Geometry check sheet. Reference: drawing and pictorial views, mm from the part's lowest x, y, z. Give positions to 0.01 mm unless a question says otherwise; leave off trailing zeros. Order: outer loops, then holes, each group sorted by start corner. A loop starts at its lowest first (then second) coordinate and runs counter-clockwise, first axis right, second up. Notation, with made-up numbers: M 35,36 L 45,36 A36 ccw 45,70 Z; hole C 89.25,-10.75 d7. An arc over 180 degrees is marked long. Use CSV: the item, a comma, the result in double quotes. Start each with the question number.
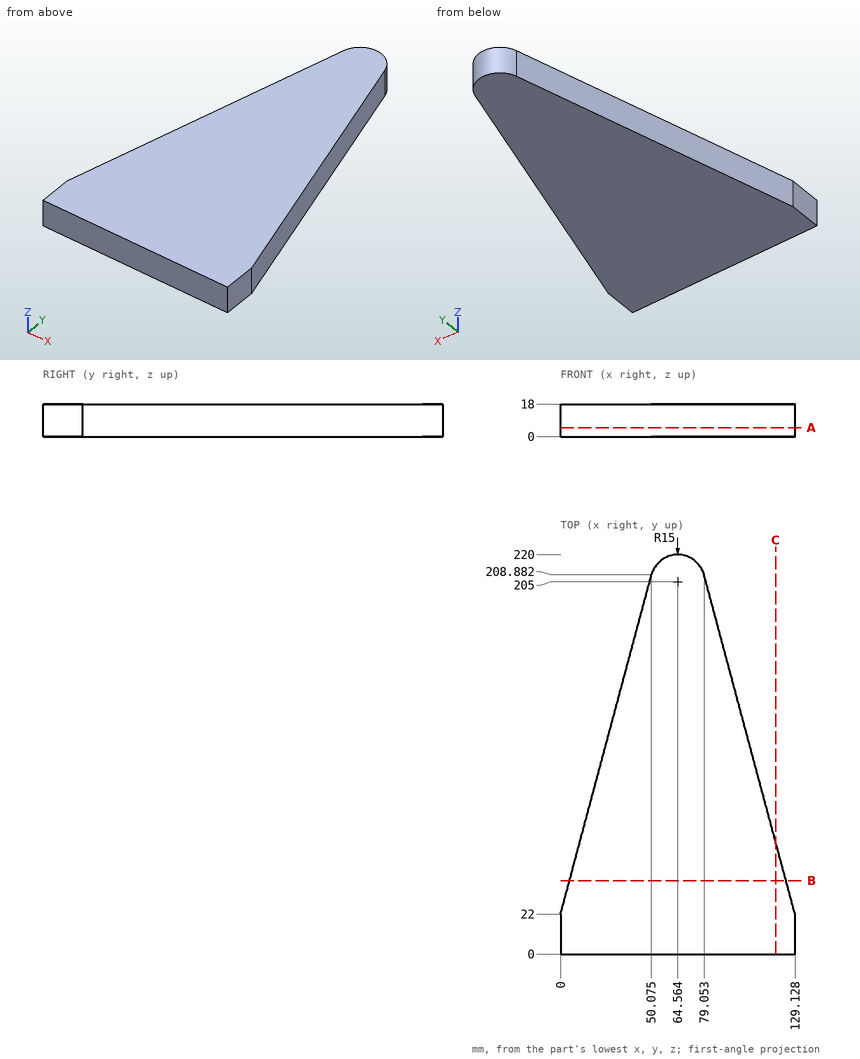
(1) Thickness scan on line 1 (X direction, y = 144, z = 14.5); line 2 (X direction, y = 35.5, z = 1.5). Record the ranges inside material, lowest first.
(2) Sectioned sample at C-C on x = 118.5. Record the cut outline in (y, z).
(3) Sectioned sample at A-A on z = 5. Record the cut outline in (x, y) (1 decimal), then the cut area to 3 significant figures.
(4) Sectioned sample at B-B on y = 40.5. Record the cut outline in (x, z), then the cut area to 3 significant figures.
(5) Go/stop test with flat-tipped pins: P1, Ø8, axis at y = 158, z = 14.5, coming from the +X side; P2, Ø10, axis at y = 143, z = 6.5, coming from the -X side. Record where each tip stops, or that it passes through.
Responses:
1,line 1,"32.69 to 96.44"
1,line 2,"3.62 to 125.51"
2,outline,"M 0,0 L 61.66,0 L 61.66,18 L 0,18 Z"
3,outline,"M 0,0 L 129.1,0 L 129.1,22 L 79.1,208.9 A15 ccw 50.1,208.9 L 0,22 Z"
3,area,"17,900 mm2"
4,outline,"M 4.96,0 L 124.17,0 L 124.17,18 L 4.96,18 Z"
4,area,"2,150 mm2"
5,P1,"x = 93.76"
5,P2,"x = 31.08"
